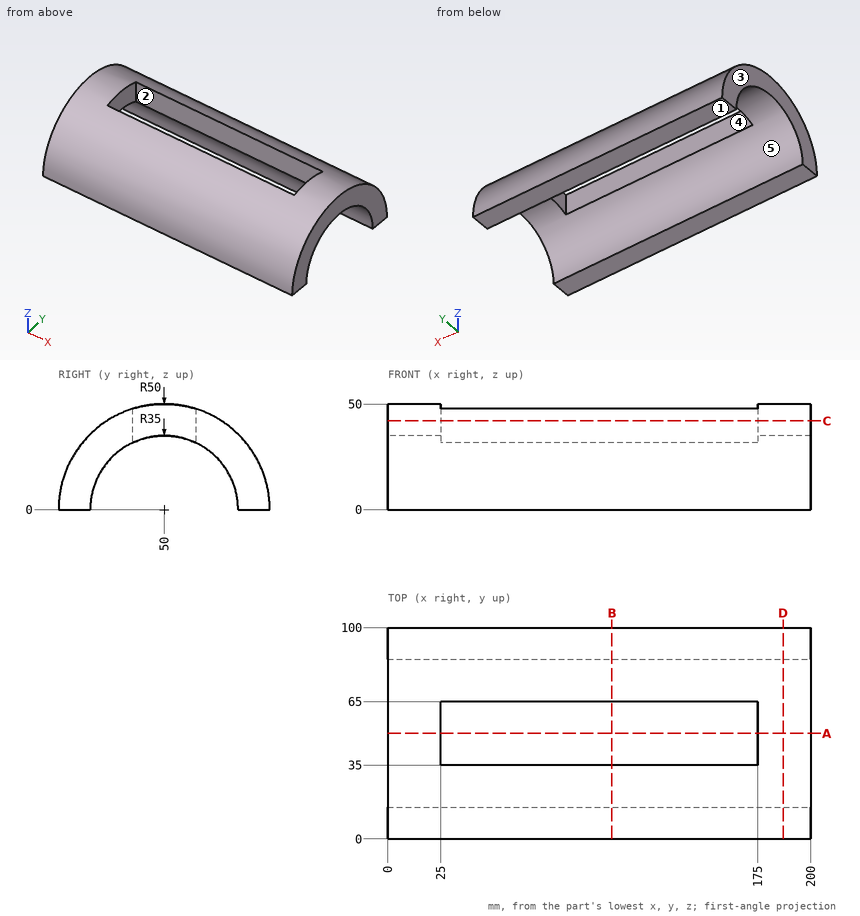
The figure shows three views and two pictorial views of one solid part (mm, origin at its lowest corner). Answer the questions. A direction names the side the tool comes from. Give positions to 0.01 mm unless a question says otherwise; leave off trailing zeros. Loops run counter-clockwise (first coordinate to the right, second up) from the corner with the lowest first, then second, coordinate; pieces in that order, holes last. Notation, with made-up numbers: (-34.75, 27.5) -> (11.25, 27.5) arc R13 cw to (11.25, 44.5) -> close; hole circle Ø7 at (-10.5, 49). An arc over 180 degrees is marked (long way). Use a Markdown table: item, result. Add a question column.
1. For the marked faces 4 and 5, determine the directions among +Z, -Z, +X, -X, +Y, -Y from which every point of the face is accessible in a straight line to the end or side of a thin tool.
2. Determine the mould class of the marked faces 1, 2 and 3 for opening direction X: released by +X, released by -X, zero draft, split by the parting line, or undercut.
3. Section B-B on x = 106 is taken. Determine the outline of the cut face in (y, z), and give its area (3 significant figures).
4. Section C-C on z = 42 is taken. Determine the outline of the cut face in (x, y), and give its area (3 significant figures).
5. Section D-D on x = 187 is taken. Determine the outline of the cut face in (y, z), and give its area (3 significant figures).
6. Flat-ended cylindrical pins translate along their axes: pin 1 Ø4 at (y, z) = (70.5, 32.5) entering from -X; pin 2 Ø2 at (x, z) = (126.5, 40.5) entering from +Y; pin 3 Ø8 at (x, z) = (83.5, 42) entering from +Y; pin 4 Ø13 at (x, z) = (77, 40) entering from -Y. Find the tip coordinate at first contact, or state that the pin passes through.
7. Section A-A on y = 50 is taken. Determine the outline of the cut face in (x, z).
8. Find the intervals of material crossed by probe 1 along X at (y, z) = (45, 41.5); probe 2 along Y at (x, z) = (162, 7); probe 3 along Y at (x, z) = (34, 36), in increasing order.
Results below:
| question | item | result |
|---|---|---|
| 1 | face 4 | +Z, -Z |
| 1 | face 5 | -Z, +X, -X |
| 2 | face 1 | zero draft |
| 2 | face 2 | undercut |
| 2 | face 3 | released by -X |
| 3 | outline | (0, 0) -> (15, 0) arc R35 cw to (35, 31.62) -> (35, 47.7) arc R50 ccw to start; (65, 31.62) arc R35 cw to (85, 0) -> (100, 0) arc R50 ccw to (65, 47.7) -> close |
| 3 | area | 1,540 mm^2 |
| 4 | outline | (0, 22.87) -> (200, 22.87) -> (200, 77.13) -> (0, 77.13) -> close; hole (25, 35) -> (175, 35) -> (175, 65) -> (25, 65) -> close |
| 4 | area | 6,350 mm^2 |
| 5 | outline | (0, 0) -> (15, 0) arc R35 cw to (85, 0) -> (100, 0) arc R50 ccw to start |
| 5 | area | 2,000 mm^2 |
| 6 | pin 1 | stops at x = 0 |
| 6 | pin 2 | stops at y = 80.66 |
| 6 | pin 3 | stops at y = 82.5 |
| 6 | pin 4 | stops at y = 12.88 |
| 7 | outline | (0, 35) -> (25, 35) -> (25, 50) -> (0, 50) -> close; (175, 35) -> (200, 35) -> (200, 50) -> (175, 50) -> close |
| 8 | probe 1 | x = 0 to 25, 175 to 200 |
| 8 | probe 2 | y = 0.49 to 15.71, 84.29 to 99.51 |
| 8 | probe 3 | y = 15.3 to 35, 65 to 84.7 |
